from build123d import *

# Parameters (mm, degrees)
SKETCH1_W           = 50
SKETCH1_H           = 50
BOSS_EXTRUDE1_DEPTH = 4
SKETCH2_W           = 4
SKETCH2_H           = 4
CUT_EXTRUDE1_DEPTH  = 4
SKETCH3_R           = 7.5
CUT_EXTRUDE2_DEPTH  = 4
FILLET1_R           = 15


with BuildPart() as part:
    # Sketch1 → Boss-Extrude1 (new body)
    with BuildSketch(Plane.XY):
        Rectangle(SKETCH1_W, SKETCH1_H)
    extrude(amount=BOSS_EXTRUDE1_DEPTH)

    # Sketch2 → Cut-Extrude1 (cut)
    with BuildSketch(Plane.XY):
        with Locations((-23, -23)):
            Rectangle(SKETCH2_W, SKETCH2_H)
        with Locations((-13, -23)):
            Rectangle(SKETCH2_W, SKETCH2_H)
        with Locations((-3, -23)):
            Rectangle(SKETCH2_W, SKETCH2_H)
        with Locations((7, -23)):
            Rectangle(SKETCH2_W, SKETCH2_H)
        with Locations((17, -23)):
            Rectangle(SKETCH2_W, SKETCH2_H)
    extrude(amount=CUT_EXTRUDE1_DEPTH, mode=Mode.SUBTRACT)

    # Sketch3 → Cut-Extrude2 (cut)
    with BuildSketch(Plane.XY):
        Circle(SKETCH3_R)
    extrude(amount=CUT_EXTRUDE2_DEPTH, mode=Mode.SUBTRACT)

    # Fillet1
    fillet1_edges = [part.edges().sort_by_distance(p)[0] for p in [
        (-25, 25, 2),
        (25, 25, 2),
    ]]
    fillet(fillet1_edges, radius=FILLET1_R)


solid = part.part
Could you check a few things on this model? Use its own coordinates, in mm. A direction names the side the tool comes from. Coordinates: 2 decimals unless noted, no trailing zeros. Write each loop counter-clockwise with the first axis right and the second up, starting at its lowest first coordinate (ties: lowest second). Pieces come first, ordered by that corner, then holes. Notation, with made-up numbers: (69.5, 65.25) - (124.5, 65.25) arc R34 ccw to (124.5, 99.25) - close; hole circle Ø4 at (58.25, 4.5). An arc over 180 degrees is marked (long way). Put each result on its own line as item: value. Start each with the question number.
Q1. Please list where these lines run through material, in increasing order: L1, parallel to X at y = -21.5, z = 3.55; L2, parallel to Y at x = 0, z = 2.8; L3, parallel to X at y = 3.5, z = 2.15.
Q2. I'm going to push flat-ended pins straight in: P1, Ø1.2, axis at x = 8, z = 1.5, coming from the -Y side; P2, Ø2, axis at y = -23, z = 1, coming from the -X side. Where does each tip first touch, or does it pass through?
Q3. I want a section at A-A on y = 0. Write out the boundary of the cut face in (x, z).
Q4. I want a section at D-D on x = -19. Write out the boundary of the cut face in (y, z).
Q5. I want a section at C-C on z = 2.8. Write out the boundary of the cut face in (x, y).
Q6. Thinking about a two-plate mould opening in X: for faces 4 (the flat face through (-3, -21, 2)), 5 (the flat face through (-25, -6, 2)), 6 (the flat face through (-18, -25, 2)), which applies, pulls with the +X half, pulls with the -X half, needs draft (parallel to the pull), parting line crosses it, or undercut?
Q7. Which directions (+Z, -Z, +X, -X, +Y, -Y) give clear straight access to the entire face, cutting with the end or side of a thin tool? Please do faces 1 (the flat face through (-5, -23, 2)), 2 (the flat face through (-21, -23, 2)), 3 (the flat face through (5, 6, 4)).
Checks:
1. L1: -21 to -15, -11 to -5, -1 to 5, 9 to 15, 19 to 25
1. L2: -25 to -7.5, 7.5 to 25
1. L3: -25 to -6.63, 6.63 to 25
2. P1: y = -21
2. P2: x = -21
3. outline: (-25, 0) - (-7.5, 0) - (-7.5, 4) - (-25, 4) - close; (7.5, 0) - (25, 0) - (25, 4) - (7.5, 4) - close
4. outline: (-25, 0) - (22, 0) - (22, 4) - (-25, 4) - close
5. outline: (-25, -21) - (-21, -21) - (-21, -25) - (-15, -25) - (-15, -21) - (-11, -21) - (-11, -25) - (-5, -25) - (-5, -21) - (-1, -21) - (-1, -25) - (5, -25) - (5, -21) - (9, -21) - (9, -25) - (15, -25) - (15, -21) - (19, -21) - (19, -25) - (25, -25) - (25, 10) arc R15 ccw to (10, 25) - (-10, 25) arc R15 ccw to (-25, 10) - close; hole circle Ø15 at (0, 0)
6. face 4: undercut
6. face 5: pulls with the -X half
6. face 6: needs draft
7. face 1: +Z, -Z, -Y
7. face 2: +Z, -Z, -X, -Y
7. face 3: +Z, +X, -X, +Y, -Y
